Model file for the job. Use its own axes, mm. Face numbers are marked on the shaded views. Coordinates: 2 decimals unless noted, no trailing zeros. Loops run counter-clockwise (first coordinate to the right, second up) from the corner with the lowest first, then second, coordinate; pieces in that order, holes last. Notation, with made-up numbers: M 50,89.25 L 73,89.25 A19 cw 73,112.25 Z; hole C 71,36 d8. An arc over 180 degrees is marked long. Write item = value, one per line. Start each with the question number.
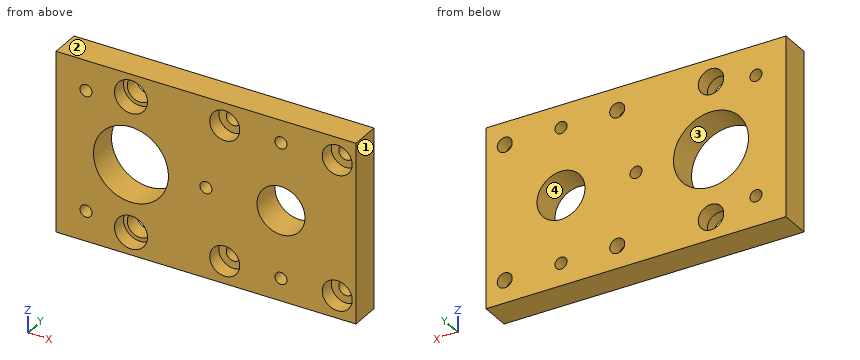
from build123d import *

# Parameters (mm, degrees)
SKETCH_1_W          = 20
SKETCH_1_H          = 12
SKETCH_1_R          = 2.5
SKETCH_1_R_2        = 1.6
EXTRUDE_1_DEPTH     = 2
SKETCH_1_4_R        = 0.5
SKETCH_1_4_R_2      = 0.85
CUT_EXTRUDE_1_DEPTH = 17.278820596
SKETCH_1_5_R        = 1
SKETCH_1_5_R_2      = 1.1
CUT_EXTRUDE_2_DEPTH = 1
SKETCH_2_R          = 0.4
CUT_EXTRUDE_3_DEPTH = 17.278820596


with BuildPart() as part:
    # 草图1 → 凸台-拉伸1 (new body)
    with BuildSketch(Plane(origin=(0, 0, 0), x_dir=(1, 0, 0), z_dir=(0, 1, 0))):
        with Locations((-5, 0)):
            Rectangle(SKETCH_1_W, SKETCH_1_H)
        with Locations(Location((-10, 0, 0), (0, 0, 270))):
            Circle(SKETCH_1_R, mode=Mode.SUBTRACT)
        with Locations(Location((0, 0, 0), (0, 0, 270))):
            Circle(SKETCH_1_R_2, mode=Mode.SUBTRACT)
    extrude(amount=EXTRUDE_1_DEPTH)

    # 草图1<4> → 切除-拉伸1 (cut, through all)
    with BuildSketch(Plane(origin=(0, 0, 0), x_dir=(1, 0, 0), z_dir=(0, 1, 0))):
        with Locations(Location((-3.75, 4.5, 0), (0, 0, 270))):
            Circle(SKETCH_1_4_R)
        with Locations(Location((3.75, -4.5, 0), (0, 0, 270))):
            Circle(SKETCH_1_4_R)
        with Locations(Location((3.75, 4.5, 0), (0, 0, 270))):
            Circle(SKETCH_1_4_R)
        with Locations(Location((-3.75, -4.5, 0), (0, 0, 270))):
            Circle(SKETCH_1_4_R)
        with Locations(Location((-10, 4.5, 0), (0, 0, 270))):
            Circle(SKETCH_1_4_R_2)
        with Locations(Location((-10, -4.5, 0), (0, 0, 270))):
            Circle(SKETCH_1_4_R_2)
    extrude(amount=CUT_EXTRUDE_1_DEPTH, mode=Mode.SUBTRACT)

    # 草图1<5> → 切除-拉伸2 (cut)
    with BuildSketch(Plane(origin=(0, 0, 0), x_dir=(1, 0, 0), z_dir=(0, 1, 0))):
        with Locations(Location((-3.75, 4.5, 0), (0, 0, 270))):
            Circle(SKETCH_1_5_R)
        with Locations(Location((3.75, 4.5, 0), (0, 0, 270))):
            Circle(SKETCH_1_5_R)
        with Locations(Location((-3.75, -4.5, 0), (0, 0, 270))):
            Circle(SKETCH_1_5_R)
        with Locations(Location((3.75, -4.5, 0), (0, 0, 270))):
            Circle(SKETCH_1_5_R)
        with Locations(Location((-10, -4.5, 0), (0, 0, 270))):
            Circle(SKETCH_1_5_R_2)
        with Locations(Location((-10, 4.5, 0), (0, 0, 270))):
            Circle(SKETCH_1_5_R_2)
    extrude(amount=CUT_EXTRUDE_2_DEPTH, mode=Mode.SUBTRACT)

    # 草图2 → 切除-拉伸3 (cut, through all)
    with BuildSketch(Plane.XZ):
        with Locations(Location((-13, 4, 0), (0, 0, 270))):
            Circle(SKETCH_2_R)
        with Locations(Location((-5, 0, 0), (0, 0, 270))):
            Circle(SKETCH_2_R)
        with Locations(Location((-13, -4, 0), (0, 0, 270))):
            Circle(SKETCH_2_R)
        with Locations(Location((0, -4.5, 0), (0, 0, 270))):
            Circle(SKETCH_2_R)
        with Locations(Location((0, 4.5, 0), (0, 0, 270))):
            Circle(SKETCH_2_R)
    extrude(amount=-CUT_EXTRUDE_3_DEPTH, mode=Mode.SUBTRACT)


solid = part.part
Item 1: Pull direction Z, two halves, no side cores. Call the marked faces 1, 2, 3 and 4: +Z half, -Z half, draft (parallel to the pull), parting line (faces both ways), or undercut.
Item 2: Pin check, flat tips, straight feed: pin 1 Ø1.2 at (x, z) = (-3.75, -4.5) entering from +Y; pin 2 Ø1.8 at (x, z) = (3.75, -4.5) entering from -Y. Stop position of each tip, or through.
Item 3: Probe L1, parallel to X at y = 1.5, z = 0; L2, parallel to Z at x = -3.75, y = 1.25; L3, parallel to X at y = 0.45, z = 4. List the from-to ranges inside material, lowest first.
Item 4: Cut at C-C (z = 0). Give the cut face in (x, y), plus the area to 3 significant figures.
Item 5: Cut at B-B (y = 1.2). Give the number of separate pieces and of enclosed holes in the cut face, plus the area to 3 significant figures.
Item 6: Cut at D-D (x = -13). Give the cut face in (y, z).
Item 7: Cut at A-A (x = 0). Give the cut face in (y, z).
Reported:
q1.face_1 = draft
q1.face_2 = +Z half
q1.face_3 = undercut
q1.face_4 = undercut
q2.pin_1 = 2
q2.pin_2 = 1
q3.L1 = -15 to -12.5, -7.5 to -5.4, -4.6 to -1.6, 1.6 to 5
q3.L2 = -6 to -5, -4 to 4, 5 to 6
q3.L3 = -15 to -13.4, -12.6 to -10.98, -9.02 to -4.62, -2.88 to 2.88, 4.62 to 5
q4.outline = M -15,0 L -12.5,0 L -12.5,2 L -15,2 Z; M -7.5,0 L -5.4,0 L -5.4,2 L -7.5,2 Z; M -4.6,0 L -1.6,0 L -1.6,2 L -4.6,2 Z; M 1.6,0 L 5,0 L 5,2 L 1.6,2 Z
q4.area = 22.0 mm^2
q5.separate_pieces = 1
q5.enclosed_holes = 13
q5.area = 202 mm^2
q6.outline = M 0,-6 L 2,-6 L 2,-4.4 L 0,-4.4 Z; M 0,-3.6 L 2,-3.6 L 2,3.6 L 0,3.6 Z; M 0,4.4 L 2,4.4 L 2,6 L 0,6 Z
q7.outline = M 0,-6 L 2,-6 L 2,-4.9 L 0,-4.9 Z; M 0,-4.1 L 2,-4.1 L 2,-1.6 L 0,-1.6 Z; M 0,1.6 L 2,1.6 L 2,4.1 L 0,4.1 Z; M 0,4.9 L 2,4.9 L 2,6 L 0,6 Z
